Verification items for the finished model (mm, model axes). Coordinates: 2 decimals unless noted, no trailing zeros. Order: outer loops, then holes, each group sorted by start corner. A loop starts at its lowest first (then second) coordinate and runs counter-clockwise, first axis right, second up. Notation, with made-up numbers: (-5, -19.75) -> (45, -19.75) arc R18 cw to (45, -4.75) -> close; hole circle Ø9 at (-20.5, 7.5). An arc over 180 degrees is marked (long way). Write item = value, one per line. Start each with the question number.
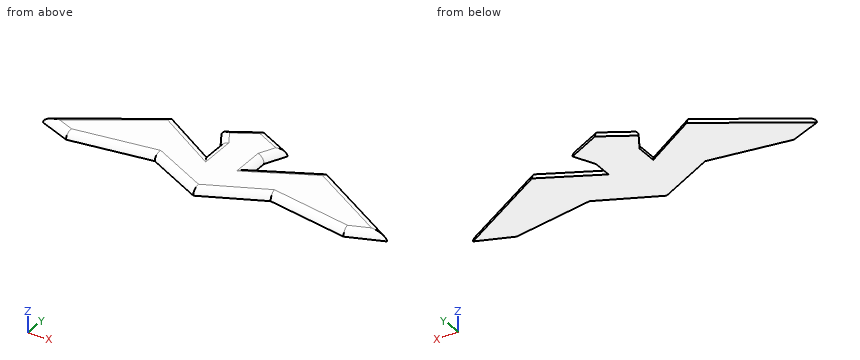
from build123d import *

# Parameters (mm, degrees)
F1_DEPTH = 2.54
F2_R     = 2.53999


# Not quite as in the source:
# - a fillet or chamfer is up to 0.001 mm smaller than in the source, because OpenCascade refuses the exact size


with BuildPart() as f1:
    # F0 (on Top) → F1 (new body)
    with BuildSketch(Plane.XY):
        Polygon((-27.0982775837, 20.9077224135), (-59.8030947149, 0), (-48.823621124, -4.3217078783), (-20.0901012868, 0), (0, -9.9282488227), (21.0245233029, 0), (49.9916523695, -4.7889198177), (62.3727589846, 0), (28.4999143332, 19.9733003974), (8.1038610589, 9.461035952), (8.1038610589, 16.395563461), (11.6802928969, 23.7109921873), (0, 29.4213576296), (-11.2130800262, 22.7765701711), (-7.4753868394, 16.4692122489), (-7.4753868394, 8.9938249439), align=None)
    extrude(amount=F1_DEPTH)

    # F2 (radius 2.54 in the source; OpenCascade refuses exactly that, so slightly less here)
    f2_edges = [f1.edges().sort_by_distance(p)[0] for p in [
        (-43.450686, 10.453861, 2.54),
        (-17.286832, 14.950774, 2.54),
        (-7.475387, 12.731519, 2.54),
        (-9.344233, 19.622891, 2.54),
        (-5.60654, 26.098964, 2.54),
        (5.840146, 26.566175, 2.54),
        (9.892077, 20.053278, 2.54),
        (8.103861, 12.9283, 2.54),
        (18.301888, 14.717168, 2.54),
        (45.436337, 9.98665, 2.54),
        (-54.313358, -2.160854, 2.54),
        (-34.456861, -2.160854, 2.54),
        (-10.045051, -4.964124, 2.54),
        (10.512262, -4.964124, 2.54),
        (35.508088, -2.39446, 2.54),
        (56.182206, -2.39446, 2.54),
    ]]
    fillet(f2_edges, radius=F2_R)


solid = f1.part
Item 1: Thickness scan on line 1 (X direction, y = 12.5, z = 0.7); line 2 (X direction, y = 17, z = 1.45); line 3 (Y direction, x = 8, z = 1.45). Record the ranges inside material, lowest first.
Item 2: Section check A-A (z = 1.15). Record the boundary of the cut face in (x, y).
Item 3: Gauge pin test, flat ends, axial feed: P1, Ø5, axis at x = -12, y = 13.5, coming from the +Z side; P2, Ø3, axis at x = 16, y = -4.5, coming from the +Z side. Record the tip position at first contact, or that the pin passes through.
Filled sheet:
q1.line_1 = -40.07 to -13.44, -7.38 to 8.01, 14.21 to 40.98
q1.line_2 = -32.37 to -21.54, -7.26 to 7.89, 23.72 to 32.65
q1.line_3 = -5.65 to 8.9, 17.22 to 25
q2.outline = (-59.2, 0.06) -> (-48.79, -4.04) -> (-20.05, 0.29) -> (0, -9.62) -> (20.98, 0.29) -> (49.96, -4.51) -> (61.74, 0.05) -> (28.49, 19.66) -> (7.83, 9.01) -> (7.83, 16.46) -> (11.31, 23.58) -> (0.01, 29.11) -> (-10.84, 22.68) -> (-7.2, 16.54) -> (-7.2, 8.5) -> (-27.09, 20.58) -> close
q3.P1 = 2.02
q3.P2 = through
